Model file for the job. Use its own axes, mm. Face numbers are marked on the shaded views. A direction names the side the tool comes from. Give positions to 0.01 mm unless a question says otherwise; leave off trailing zeros. Write each loop counter-clockwise with the first axis right and the second up, starting at its lowest first coordinate (ties: lowest second). Pieces come first, ordered by that corner, then holes.
```python
from build123d import *


with BuildPart() as f1:
    # F0 (on Front) → F1 (revolve)
    with BuildSketch(Plane.XZ):
        Polygon((60, 80), (40, 80), (40, 72), (25, 72), (25, 8), (40, 8), (40, 0), (60, 0), (60, 34), (59, 34), (58, 35.5), (58, 36.5), (55, 36.5), (55, 43.5), (58, 43.5), (58, 44.5), (59, 46), (60, 46), align=None)
    revolve(axis=Axis((0, 0, 40), (0, 0, 1)))


solid = f1.part
```
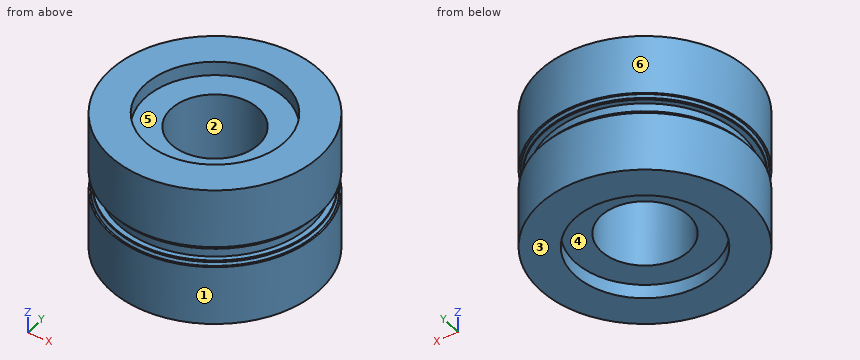
1. Which spindle directions (+Z, -Z, +X, -X, +Y, -Y) get a long thin tool onto all of the face, cutting with end or side? Do the marked faces 4, 5 and 6. Say none if no direction does.
Calculated:
face 4: -Z
face 5: +Z
face 6: +Z, -Z
2. Pin check, flat tips, straight feed: P1, Ø10, axis at x = 42.5, z = 51, coming from the +Y side; P2, Ø24, axis at x = 16, y = 13, coming from the +Z side; P3, Ø3, axis at x = 22, y = -29.5, coming from the -Z side. Stop position of each tip, or through.
Calculated:
P1: stops at y = 46.84
P2: stops at z = 72
P3: stops at z = 8
3. Probe probe 1 along Z at (x, y) = (-21.5, 55.5); probe 2 along Y at (x, z) = (0, 1); probe 3 along Z at (x, y) = (32.5, -11). List the from-to ranges inside material, lowest first.
Calculated:
probe 1: z = 0 to 34, 46 to 80
probe 2: y = -60 to -40, 40 to 60
probe 3: z = 8 to 72
4. Slice it at A-A, the plane z = 62. Write the cut outline in (x, y).
Calculated:
outline: circle Ø120 at (0, 0); hole circle Ø50 at (0, 0)
5. Pull direction X, two halves, no side cores. Call the marked faces 1, 2 and 3: +X half, -X half, draft (parallel to the pull), parting line (faces both ways), or undercut.
Calculated:
face 1: parting line
face 2: undercut
face 3: draft
